from build123d import *

# Parameters (mm, degrees)
CUT_EXTRUDE1_DEPTH      = 11.43
SKETCH3_R               = 3.175
CUT_EXTRUDE2_DEPTH      = 52.61889964
CUT_EXTRUDE3_DEPTH      = 50.121262199
CUT_EXTRUDE3_DEPTH_BACK = 50.121262199
SKETCH4_W               = 5.08
SKETCH4_H               = 1.27
FILLET1_R               = 1.905


with BuildPart() as part:
    # Sketch1 → Revolve1 (revolve)
    with BuildSketch(Plane.XY, mode=Mode.PRIVATE) as revolve1_sk:
        with BuildLine():
            Line((0, 0), (0, 5.602635041))
            Line((0, 5.602635041), (-2.54, 5.602635041))
            Line((-2.54, 5.602635041), (-2.54, 38.1))
            Line((-2.54, 38.1), (0, 38.1))
            Line((0, 38.1), (0, 45.72))
            ThreePointArc((0, 45.72), (-8.980256121, 42.000256121), (-12.7, 33.02))
            Line((-12.7, 33.02), (-12.7, 0))
            Line((-12.7, 0), (0, 0))
        make_face()
    revolve(revolve1_sk.sketch.rotate(Axis((0, 0, 0), (0, 1, 0)), 270), axis=Axis((0, 0, 0), (0, 1, 0)))

    # Sketch2 → Cut-Extrude1 (cut)
    with BuildSketch(Plane.XZ):
        with BuildLine():
            Line((-2.54, 12.443407893), (-2.54, -12.443407893))
            ThreePointArc((-2.54, -12.443407893), (0, -12.7), (2.54, -12.443407893))
            Line((2.54, -12.443407893), (2.54, 12.443407893))
            ThreePointArc((2.54, 12.443407893), (0, 12.7), (-2.54, 12.443407893))
        make_face()
        with BuildLine():
            Line((-7.62, 10.16), (-7.62, -10.16))
            ThreePointArc((-7.62, -10.16), (-12.7, 0), (-7.62, 10.16))
        make_face()
        with BuildLine():
            Line((7.62, 10.16), (7.62, -10.16))
            ThreePointArc((7.62, -10.16), (12.7, 0), (7.62, 10.16))
        make_face()
    extrude(amount=-CUT_EXTRUDE1_DEPTH, mode=Mode.SUBTRACT)

    # Sketch3 → Cut-Extrude2 (cut, through all)
    with BuildSketch(Plane.ZY.offset(7.62)):
        with Locations((0, 5.08)):
            Circle(SKETCH3_R)
        with BuildLine():
            Line((0, 0), (-12.443407893, 0))
            Line((-12.443407893, 0), (-12.443407893, 11.43))
            Line((-12.443407893, 11.43), (-3.796422114, 1.704562379))
            ThreePointArc((-3.796422114, 1.704562379), (-2.080766311, 0.445691901), (0, 0))
        make_face()
    extrude(amount=-CUT_EXTRUDE2_DEPTH, mode=Mode.SUBTRACT)

    # Sketch4 → Cut-Extrude3 (cut, two sides: drawn at the far end of the back side and taken through both)
    with BuildSketch(Plane.XY.offset(-CUT_EXTRUDE3_DEPTH_BACK)):
        with Locations((0, 32.385)):
            Rectangle(SKETCH4_W, SKETCH4_H)
        with Locations((0, 37.465)):
            Rectangle(SKETCH4_W, SKETCH4_H)
    extrude(amount=CUT_EXTRUDE3_DEPTH + CUT_EXTRUDE3_DEPTH_BACK, mode=Mode.SUBTRACT)

    # Fillet1
    # the kernel refuses this fillet: 1.905 mm, written as the material it takes off along each edge
    with BuildSketch(Plane(origin=(0, 33.02, 0), x_dir=(-0.60062876969462, 0, 0.7995280364159391), z_dir=(-0.7995280364159391, 0, -0.60062876969462))) as fillet1_piece_1_section:
        with BuildLine():
            CenterArc((10.625582337, 1.905), FILLET1_R, 270, 100.164248622)
            Line((10.625582337, 0), (12.7, 0))
            ThreePointArc((12.7, 0), (12.650073138, 1.125010933), (12.500685102, 2.241176471))
        make_face()
    fillet1_piece_1 = revolve(axis=Axis((0, 33.02, 0), (0, 1, 0)), revolution_arc=73.829886486, mode=Mode.PRIVATE)
    fillet1_piece_1 = split(fillet1_piece_1, bisect_by=Plane(origin=(2.54, 33.536908465, 12.1243087), z_dir=(-1, 0, 0)), keep=Keep.TOP, mode=Mode.PRIVATE)
    fillet1_piece_1 = split(fillet1_piece_1, bisect_by=Plane(origin=(-2.54, 33.536908465, 12.1243087), z_dir=(1, 0, 0)), keep=Keep.TOP, mode=Mode.PRIVATE)
    add(fillet1_piece_1, mode=Mode.SUBTRACT)
    with BuildSketch(Plane(origin=(0, 36.83, 0), x_dir=(0.5180820301307626, 0, 0.8553309359865265), z_dir=(0.8553309359865265, 0, -0.5180820301307626))) as fillet1_piece_2_section:
        with BuildLine():
            CenterArc((10.625582337, 1.905), FILLET1_R, 270, 79.835751378)
            Line((10.625582337, 0), (12.115027858, 0))
            ThreePointArc((12.115027858, 0), (12.332827452, 0.778273257), (12.500685102, 1.568823529))
        make_face()
    fillet1_piece_2 = revolve(axis=Axis((0, 36.83, 0), (0, -1, 0)), revolution_arc=62.407371172, mode=Mode.PRIVATE)
    fillet1_piece_2 = split(fillet1_piece_2, bisect_by=Plane(origin=(2.54, 36.48222625, 11.799196002), z_dir=(-1, 0, 0)), keep=Keep.TOP, mode=Mode.PRIVATE)
    fillet1_piece_2 = split(fillet1_piece_2, bisect_by=Plane(origin=(-2.54, 36.48222625, 11.799196002), z_dir=(1, 0, 0)), keep=Keep.TOP, mode=Mode.PRIVATE)
    add(fillet1_piece_2, mode=Mode.SUBTRACT)
    with BuildSketch(Plane(origin=(0, 36.83, 0), x_dir=(-0.5180758180945624, 0, -0.8553346986447176), z_dir=(-0.8553346986447176, 0, 0.5180758180945624))) as fillet1_piece_3_section:
        with BuildLine():
            CenterArc((10.625582337, 1.905), FILLET1_R, 270, 79.835751378)
            Line((10.625582337, 0), (12.115027858, 0))
            ThreePointArc((12.115027858, 0), (12.332827452, 0.778273257), (12.500685102, 1.568823529))
        make_face()
    fillet1_piece_3 = revolve(axis=Axis((0, 36.83, 0), (0, -1, 0)), revolution_arc=31.203269463, mode=Mode.PRIVATE)
    fillet1_piece_3 = split(fillet1_piece_3, bisect_by=Plane(origin=(-2.54, 36.482226182, -11.799196273), z_dir=(1, 0, 0)), keep=Keep.TOP, mode=Mode.PRIVATE)
    add(fillet1_piece_3, mode=Mode.SUBTRACT)
    with BuildSketch(Plane(origin=(0, 33.02, 0), x_dir=(0.6006217587640166, 0, -0.7995333031833131), z_dir=(0.7995333031833131, 0, 0.6006217587640166))) as fillet1_piece_4_section:
        with BuildLine():
            CenterArc((10.625582337, 1.905), FILLET1_R, 270, 100.164248622)
            Line((10.625582337, 0), (12.7, 0))
            ThreePointArc((12.7, 0), (12.650073138, 1.125010933), (12.500685102, 2.241176471))
        make_face()
    fillet1_piece_4 = revolve(axis=Axis((0, 33.02, 0), (0, 1, 0)), revolution_arc=36.914440828, mode=Mode.PRIVATE)
    fillet1_piece_4 = split(fillet1_piece_4, bisect_by=Plane(origin=(2.54, 33.536908471, -12.124308945), z_dir=(-1, 0, 0)), keep=Keep.TOP, mode=Mode.PRIVATE)
    add(fillet1_piece_4, mode=Mode.SUBTRACT)
    with BuildSketch(Plane(origin=(0, 33.02, 0), x_dir=(0, 0, -1), z_dir=(1, 0, 0))) as fillet1_piece_5_section:
        with BuildLine():
            CenterArc((10.625582337, 1.905), FILLET1_R, 270, 100.164248622)
            Line((10.625582337, 0), (12.7, 0))
            ThreePointArc((12.7, 0), (12.650073138, 1.125010933), (12.500685102, 2.241176471))
        make_face()
    fillet1_piece_5 = revolve(axis=Axis((0, 33.02, 0), (0, 1, 0)), revolution_arc=36.914440828, mode=Mode.PRIVATE)
    fillet1_piece_5 = split(fillet1_piece_5, bisect_by=Plane(origin=(-2.54, 33.536908442, -12.124308642), z_dir=(1, 0, 0)), keep=Keep.TOP, mode=Mode.PRIVATE)
    add(fillet1_piece_5, mode=Mode.SUBTRACT)
    with BuildSketch(Plane(origin=(0, 36.83, 0), x_dir=(0, 0, -1), z_dir=(-1, 0, 0))) as fillet1_piece_6_section:
        with BuildLine():
            CenterArc((10.625582337, 1.905), FILLET1_R, 270, 79.835751378)
            Line((10.625582337, 0), (12.115027858, 0))
            ThreePointArc((12.115027858, 0), (12.332827452, 0.778273257), (12.500685102, 1.568823529))
        make_face()
    fillet1_piece_6 = revolve(axis=Axis((0, 36.83, 0), (0, -1, 0)), revolution_arc=31.203269463, mode=Mode.PRIVATE)
    fillet1_piece_6 = split(fillet1_piece_6, bisect_by=Plane(origin=(2.54, 36.482226255, -11.799195907), z_dir=(-1, 0, 0)), keep=Keep.TOP, mode=Mode.PRIVATE)
    add(fillet1_piece_6, mode=Mode.SUBTRACT)


solid = part.part
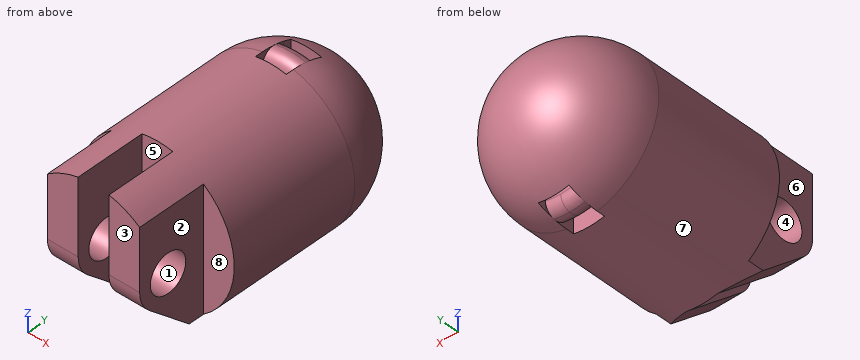
The model under review builds one solid part; all positions refer to its coordinate system, in mm. Face numbers are marked on the shaded views. A direction names the side the tool comes from. Coordinates: 2 decimals unless noted, no trailing zeros. Write each loop counter-clockwise with the first axis right and the second up, starting at its lowest first coordinate (ties: lowest second). Pieces come first, ordered by that corner, then holes. Notation, with made-up numbers: (53, 59) -> (60, 59) arc R21 cw to (60, 65) -> close; hole circle Ø4 at (84, -27). An arc over 180 degrees is marked (long way). Answer in a Markdown table with one row per item.
1. We need section B-B, the plane y = 23.5. State the section outline as (x, z) points, and give its area (3 significant figures).
Answers below:
| item | result |
|---|---|
| outline | circle Ø25.4 at (0, 0); hole circle Ø5.08 at (0, 0) |
| area | 486 mm^2 |
2. We need section D-D, the plane x = 2. Give the number of separate pieces and of enclosed holes in the cut face, and give its area (3 significant figures).
Answers below:
| item | result |
|---|---|
| separate pieces | 5 |
| enclosed holes | 0 |
| area | 648 mm^2 |
3. We need section A-A, the plane z = 4.25. State the section outline as (x, y) points, and give its area (3 significant figures).
Answers below:
| item | result |
|---|---|
| outline | (-11.97, 11.43) -> (-7.62, 11.43) -> (-7.62, 0) -> (-2.54, 0) -> (-2.54, 11.43) -> (2.54, 11.43) -> (2.54, 0) -> (7.62, 0) -> (7.62, 11.43) -> (11.97, 11.43) -> (11.97, 33.02) arc R11.97 ccw to (-11.97, 33.02) -> close; hole (-2.54, 31.75) -> (2.54, 31.75) -> (2.54, 33.02) -> (-2.54, 33.02) -> close; hole (-2.54, 36.83) -> (2.54, 36.83) -> (2.54, 38.1) -> (-2.54, 38.1) -> close |
| area | 845 mm^2 |
4. We need section C-C, the plane y = 5.08. State the section outline as (x, z) points (3 decimals).
Answers below:
| item | result |
|---|---|
| outline | (-7.62, -6.798) -> (-2.54, -6.798) -> (-2.54, -3.175) -> (-7.62, -3.175) -> close; (-7.62, 3.175) -> (-2.54, 3.175) -> (-2.54, 12.443) arc R12.7 ccw to (-7.62, 10.16) -> close; (2.54, -6.798) -> (7.62, -6.798) -> (7.62, -3.175) -> (2.54, -3.175) -> close; (2.54, 3.175) -> (7.62, 3.175) -> (7.62, 10.16) arc R12.7 ccw to (2.54, 12.443) -> close |
5. Draft analysis for pull direction Y (two halves, no side actions). For the marked faces 1, 2, 3 and 4, state which applies: +Y half, -Y half, draft (parallel to the pull), parting line (faces both ways), or undercut.
Answers below:
| item | result |
|---|---|
| face 1 | undercut |
| face 2 | draft |
| face 3 | -Y half |
| face 4 | undercut |
6. For the marked faces 5, 6, 7 and 8, list the 3-axis set-ups (+Z, -Z, +X, -X, +Y, -Y) from which the entire face can be reached by the end or side of a thin tool; tool diameter is ignored.
Answers below:
| item | result |
|---|---|
| face 5 | +Z, -Z, -Y |
| face 6 | +Z, -Z, -X, -Y |
| face 7 | +Y, -Y |
| face 8 | +Z, -Z, +X, -Y |
7. Clearance check with flat-ended pins moving along their axes: pin 1 Ø1.5 at (x, z) = (0, -6) entering from -Y; pin 2 Ø5 at (y, z) = (28.5, -1.5) entering from +X; pin 3 Ø9 at (y, z) = (6, -3) entering from +X; pin 4 Ø0.5 at (y, z) = (36, 11) entering from -X. State where each tip first meets the part, or that it passes through.
Answers below:
| item | result |
|---|---|
| pin 1 | stops at y = 11.43 |
| pin 2 | stops at x = 12.7 |
| pin 3 | stops at x = 7.62 |
| pin 4 | stops at x = -6.09 |
8. Wall thickness on probe 1 along X at (y, z) = (9, 1); probe 2 along Y at (x, z) = (0.75, -8.5); probe 3 along Y at (x, z) = (5.95, 0) (3 decimals): over which ranges is each line inside the solid? List them lowest first. Write a range as [from, to].
Answers below:
| item | result |
|---|---|
| probe 1 | x = [-7.62, -2.54], [2.54, 7.62] |
| probe 2 | y = [11.43, 31.75], [33.02, 36.83], [38.1, 42.43] |
| probe 3 | y = [0, 1.905], [8.255, 44.24] |
